Input: part model. Units: mm. Frame: model coordinates. Face numbers are marked on the shaded views. Give positions to 0.01 mm unless a question says otherwise; leave off trailing zeros. Order: outer loops, then holes, each group sorted by start corner. A loop starts at its lowest first (then second) coordinate and runs counter-clockwise, first axis right, second up. Notation, with made-up numbers: (-29.75, -30) -> (-9.75, -30) arc R11 cw to (-9.75, -16) -> close; hole circle Ø8 at (-25, 35). An arc over 180 degrees is marked (long way). Use a Markdown table: item, result. Add a question column.
from build123d import *

# Parameters (mm, degrees)
SKETCH1_W           = 300
SKETCH1_H           = 100
BOSS_EXTRUDE1_DEPTH = 5
BOSS_EXTRUDE2_DEPTH = 1


with BuildPart() as part:
    # Sketch1 → Boss-Extrude1 (new body)
    with BuildSketch(Plane(origin=(0, 0, 0), x_dir=(1, 0, 0), z_dir=(0, 1, 0))):
        Rectangle(SKETCH1_W, SKETCH1_H)
    extrude(amount=BOSS_EXTRUDE1_DEPTH)

    # Sketch2 → Boss-Extrude2 (add)
    with BuildSketch(Plane(origin=(0, 5, 0), x_dir=(1, 0, 0), z_dir=(0, 1, 0))):
        with BuildLine():
            Line((-85, 50), (-79.9507281, 14.299791972))
            ThreePointArc((-79.9507281, 14.299791972), (-75, 10), (-70.0492719, 14.299791972))
            Line((-70.0492719, 14.299791972), (-65, 50))
            Line((-65, 50), (-85, 50))
        make_face()
        with BuildLine():
            Line((70.0492719, 14.299791972), (65, 50))
            Line((65, 50), (85, 50))
            Line((85, 50), (79.9507281, 14.299791972))
            ThreePointArc((79.9507281, 14.299791972), (75, 10), (70.0492719, 14.299791972))
        make_face()
        with BuildLine():
            Line((4.957983551, -11.353162223), (10, -50))
            Line((10, -50), (-10, -50))
            Line((-10, -50), (-4.957983551, -11.353162223))
            ThreePointArc((-4.957983551, -11.353162223), (0, -7), (4.957983551, -11.353162223))
        make_face()
    extrude(amount=BOSS_EXTRUDE2_DEPTH)


solid = part.part
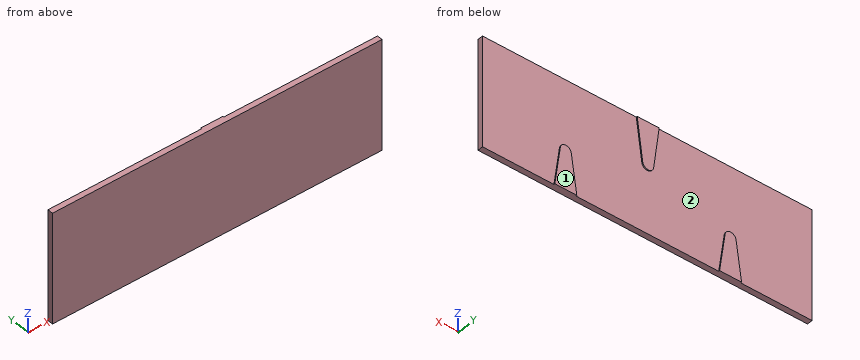
Q1. Section query D-D (x = -94.5). Return loops of the section in (y, z).
Q2. First-contact query: pin 1 (1 mm diameter, centred on x = 72, z = 13, fed in from +Y). Flat tip, straight axial feed; report the tip coordinate or a pass-through.
Q3. Section query C-C (z = 14). Return loops of the section in (x, y), plus the area to 3 significant figures.
Q4. Ray query, line 1 (Y direction, x = -46, z = -15.5); line 2 (X direction, y = 5.3, z = 25.5); line 3 (Z direction, x = -1.5, y = 5.35). Return the intervals inside material, ascending.
Q5. Section query B-B (z = 44). Return loops of the section in (x, y).
Q6. Draft query along X for the marked faces 1 and 2. Return one class per face: +X half, -X half, draft (parallel to the pull), parting line (faces both ways), or undercut.
Q7. Section query A-A (x = 75). Return loops of the section in (y, z), plus the area to 3 significant figures.
Solution:
| question | item | result |
|---|---|---|
| 1 | outline | (0, -50) -> (5, -50) -> (5, 50) -> (0, 50) -> close |
| 2 | pin 1 | stops at y = 5 |
| 3 | outline | (-150, 0) -> (150, 0) -> (150, 5) -> (5.3, 5) -> (5.3, 6) -> (-5.3, 6) -> (-5.3, 5) -> (-150, 5) -> close |
| 3 | area | 1,510 mm² |
| 4 | line 1 | y = 0 to 5 |
| 4 | line 2 | x = -6.8 to 6.8 |
| 4 | line 3 | z = 7.23 to 50 |
| 5 | outline | (-150, 0) -> (150, 0) -> (150, 5) -> (9.22, 5) -> (9.22, 6) -> (-9.22, 6) -> (-9.22, 5) -> (-150, 5) -> close |
| 6 | face 1 | draft |
| 6 | face 2 | undercut |
| 7 | outline | (0, -50) -> (6, -50) -> (6, -10) -> (5, -10) -> (5, 50) -> (0, 50) -> close |
| 7 | area | 540 mm² |
